Build history of the part. All positions in model axes, mm. Face numbers are marked on the shaded views. A direction names the side the tool comes from. Round coordinates to 2 decimals unless told otherwise and drop trailing zeros. Loops run counter-clockwise (first coordinate to the right, second up) from the corner with the lowest first, then second, coordinate; pieces in that order, holes last.
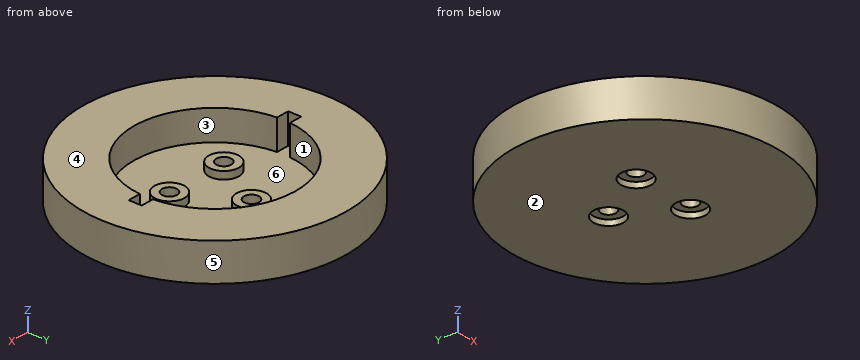
from build123d import *

# Parameters (mm, degrees)
SKETCH_1_R          = 35
EXTRUDE_1_DEPTH     = 10
CUT_EXTRUDE_1_DEPTH = 8
SKETCH_4_R          = 4
CUT_EXTRUDE_2_DEPTH = 1.5
SKETCH_6_R          = 2
CUT_EXTRUDE_3_DEPTH = 51.222007128
SKETCH_7_R          = 4
SKETCH_7_R_2        = 2
EXTRUDE_2_DEPTH     = 2
SKETCH_8_R          = 4
SKETCH_8_R_2        = 2
EXTRUDE_3_DEPTH     = 2
SKETCH_9_R          = 4
SKETCH_9_R_2        = 2
EXTRUDE_4_DEPTH     = 2


with BuildPart() as part:
    # 草图1 → 凸台-拉伸1 (new body)
    with BuildSketch(Plane.XY):
        Circle(SKETCH_1_R)
    extrude(amount=EXTRUDE_1_DEPTH)

    # 草图2 → 切除-拉伸1 (cut)
    with BuildSketch(Plane.XY.offset(10)):
        with BuildLine():
            ThreePointArc((21.428660714, 1.75), (0, 21.5), (-21.428660714, 1.75))
            Line((-21.428660714, 1.75), (-24.9, 1.75))
            Line((-24.9, 1.75), (-24.9, -1.75))
            Line((-24.9, -1.75), (-21.428660714, -1.75))
            ThreePointArc((-21.428660714, -1.75), (0, -21.5), (21.428660714, -1.75))
            Line((21.428660714, -1.75), (24.9, -1.75))
            Line((24.9, -1.75), (24.9, 1.75))
            Line((24.9, 1.75), (21.428660714, 1.75))
        make_face()
    extrude(amount=-CUT_EXTRUDE_1_DEPTH, mode=Mode.SUBTRACT)

    # 草图4 → 切除-拉伸2 (cut)
    with BuildSketch(Plane(origin=(0, 0, 0), x_dir=(-1, 0, 0), z_dir=(0, 0, -1))):
        with Locations((8.487048957, -4.9)):
            Circle(SKETCH_4_R)
        with Locations((-8.487048957, -4.9)):
            Circle(SKETCH_4_R)
        with Locations((0, 9.8)):
            Circle(SKETCH_4_R)
    extrude(amount=-CUT_EXTRUDE_2_DEPTH, mode=Mode.SUBTRACT)

    # 草图6 → 切除-拉伸3 (cut, through all)
    with BuildSketch(Plane(origin=(0, 0, 1.5), x_dir=(-1, 0, 0), z_dir=(0, 0, -1))):
        with Locations((0, 9.8)):
            Circle(SKETCH_6_R)
        with Locations((8.487048957, -4.9)):
            Circle(SKETCH_6_R)
        with Locations((-8.487048957, -4.9)):
            Circle(SKETCH_6_R)
    extrude(amount=-CUT_EXTRUDE_3_DEPTH, mode=Mode.SUBTRACT)

    # 草图7 → 凸台-拉伸2 (add)
    with BuildSketch(Plane.XY.offset(2)):
        with Locations(Location((0, 9.8, 0), (0, 0, 180))):
            Circle(SKETCH_7_R)
        with Locations(Location((0, 9.8, 0), (0, 0, 180))):
            Circle(SKETCH_7_R_2, mode=Mode.SUBTRACT)
    extrude(amount=EXTRUDE_2_DEPTH)

    # 草图8 → 凸台-拉伸3 (add)
    with BuildSketch(Plane.XY.offset(2)):
        with Locations(Location((-8.487048957, -4.9, 0), (0, 0, 180))):
            Circle(SKETCH_8_R)
        with Locations(Location((-8.487048957, -4.9, 0), (0, 0, 180))):
            Circle(SKETCH_8_R_2, mode=Mode.SUBTRACT)
    extrude(amount=EXTRUDE_3_DEPTH)

    # 草图9 → 凸台-拉伸4 (add)
    with BuildSketch(Plane.XY.offset(2)):
        with Locations(Location((8.487048957, -4.9, 0), (0, 0, 180))):
            Circle(SKETCH_9_R)
        with Locations(Location((8.487048957, -4.9, 0), (0, 0, 180))):
            Circle(SKETCH_9_R_2, mode=Mode.SUBTRACT)
    extrude(amount=EXTRUDE_4_DEPTH)


solid = part.part
(1) Slice it at C-C on y = 0. List the corners of the cut face in (x, z), plus the area to 3 significant figures.
Responses:
outline: (-35, 0) - (35, 0) - (35, 10) - (24.9, 10) - (24.9, 2) - (-24.9, 2) - (-24.9, 10) - (-35, 10) - close
area: 302 mm2
(2) Pull direction X, two halves, no side cores. Call the marked faces 3, 4, 5 and 6: +X half, -X half, draft (parallel to the pull), parting line (faces both ways), or undercut.
Responses:
face 3: undercut
face 4: draft
face 5: parting line
face 6: undercut
(3) Which spindle directions (+Z, -Z, +X, -X, +Y, -Y) get a long thin tool onto all of the face, cutting with end or side? Do the marked faces 1 and 2. Say none if no direction does.
Responses:
face 1: +Z
face 2: -Z, +X, -X, +Y, -Y
(4) Slice it at A-A on x = 0. List the corners of the cut face in (y, z).
Responses:
outline: (-35, 0) - (5.8, 0) - (5.8, 1.5) - (7.8, 1.5) - (7.8, 4) - (5.8, 4) - (5.8, 2) - (-21.5, 2) - (-21.5, 10) - (-35, 10) - close; (11.8, 1.5) - (13.8, 1.5) - (13.8, 0) - (35, 0) - (35, 10) - (21.5, 10) - (21.5, 2) - (13.8, 2) - (13.8, 4) - (11.8, 4) - close
(5) Pin check, flat tips, straight feed: P1, Ø5, axis at y = -20, z = 5, coming from the -X side; P2, Ø6.5, axis at x = 7, y = -5, coming from the +Z side; P3, Ø3, axis at x = 23.5, z = 5.5, coming from the +Y side. Stop position of each tip, or through.
Responses:
P1: stops at x = -30.31
P2: stops at z = 4
P3: stops at y = 27.22
(6) Probe line 1 (Z direction, x = 23.5, y = -1); line 2 (X direction, y = 9, z = 7); line 3 (Y direction, x = 13, z = 9.25). List the from-to ranges inside material, lowest first.
Responses:
line 1: z = 0 to 2
line 2: x = -33.82 to -19.53, 19.53 to 33.82
line 3: y = -32.5 to -17.12, 17.12 to 32.5
(7) Slice it at D-D on y = 9.8. List the corners of the cut face in (x, z).
Responses:
outline: (-33.6, 0) - (-4, 0) - (-4, 1.5) - (-2, 1.5) - (-2, 4) - (-4, 4) - (-4, 2) - (-19.14, 2) - (-19.14, 10) - (-33.6, 10) - close; (2, 1.5) - (4, 1.5) - (4, 0) - (33.6, 0) - (33.6, 10) - (19.14, 10) - (19.14, 2) - (4, 2) - (4, 4) - (2, 4) - close
(8) Slice it at B-B on z = 6.5. List the corners of the cut face in (x, y), plus the area to 3 significant figures.
Responses:
outline: circle Ø70 at (0, 0); hole (-24.9, -1.75) - (-21.43, -1.75) arc R21.5 ccw to (21.43, -1.75) - (24.9, -1.75) - (24.9, 1.75) - (21.43, 1.75) arc R21.5 ccw to (-21.43, 1.75) - (-24.9, 1.75) - close
area: 2,370 mm2
